Autodesk Inventor part; units mm, degrees
ref_plane "Work Plane1" through (6, 0, -16) normal (0, 0, -1) x (-1, 0, 0)
ref_plane "YZ Plane" through (0, 0, 0) normal (1, 0, 0) x (0, 1, 0)
ref_plane "XZ Plane" through (0, 0, 0) normal (0, 1, 0) x (-1, 0, 0)
sketch "Sketch1" plane through (0, 0, 0) normal (0, 1, 0) x (-1, 0, 0)
  line L0 (6, 8) -> (-6, 8)
  line L1 (-8, 6) -> (-8, -6)
  line L2 (-6, -8) -> (6, -8)
  line L3 (8, -6) -> (8, 6)
  arc A0 (8, 6) -> (6, 8) centre (6, 6) ccw
  arc A1 (-6, 8) -> (-8, 6) centre (-6, 6) ccw
  arc A2 (-8, -6) -> (-6, -8) centre (-6, -6) ccw
  arc A3 (6, -8) -> (8, -6) centre (6, -6) ccw
  point P0 (0, 0)
  point P1 (8, 8)
  point P2 (-8, 8)
  point P3 (8, -8)
  dimension "d0" = 16
  dimension "d1" = 16
  dimension "d2" = 8
  dimension "d3" = 8
  dimension "d4" = 2
extrude "Extrusion1" add sketch "Sketch1" along normal blind 150
sketch "Sketch2" plane through (0, 0, 0) normal (0, -1, 0) x (1, 0, 0)
  line L0 (-6, 5.875) -> (-6, 3.125) construction
  line L1 (-7.375, 5.875) -> (-7.375, 3.125)
  line L2 (-4.625, 3.125) -> (-4.625, 5.875)
  arc A0 (-4.625, 5.875) -> (-7.375, 5.875) centre (-6, 5.875) ccw
  arc A1 (-7.375, 3.125) -> (-4.625, 3.125) centre (-6, 3.125) ccw
  line L3 (6, -3.125) -> (6, -5.875) construction
  line L4 (4.625, -3.125) -> (4.625, -5.875)
  line L5 (7.375, -5.875) -> (7.375, -3.125)
  arc A2 (7.375, -3.125) -> (4.625, -3.125) centre (6, -3.125) ccw
  arc A3 (4.625, -5.875) -> (7.375, -5.875) centre (6, -5.875) ccw
  point P0 (0, 0)
  point P1 (0, 0)
  point P2 (-6, 4.5)
  point P3 (6, -4.5)
  dimension "d7" = 2.75
  dimension "d8" = 12
  dimension "d9" = 6
  dimension "d10" = 9
  dimension "d11" = 4.5
  dimension "d12" = 2.75
  dimension "d13" = 2.75
  dimension "d14" = 2.75
extrude "Extrusion2" cut sketch "Sketch2" against normal blind 2.5
sketch "Sketch3" plane through (0, 150, 0) normal (0, 1, 0) x (1, 0, 0)
  line L0 (-6, 9.5) -> (-6, 6.5) construction
  line L1 (-6.6, 9.5) -> (-6.6, 6.5)
  line L2 (-5.4, 6.5) -> (-5.4, 9.5)
  arc A0 (-5.4, 9.5) -> (-6.6, 9.5) centre (-6, 9.5) ccw
  arc A1 (-6.6, 6.5) -> (-5.4, 6.5) centre (-6, 6.5) ccw
  line L3 (6, 9.5) -> (6, 6.5) construction
  line L4 (5.4, 9.5) -> (5.4, 6.5)
  line L5 (6.6, 6.5) -> (6.6, 9.5)
  arc A2 (6.6, 9.5) -> (5.4, 9.5) centre (6, 9.5) ccw
  arc A3 (5.4, 6.5) -> (6.6, 6.5) centre (6, 6.5) ccw
  line L6 (-6, 8) -> (6, 8) construction
  line L7 (6, 8) -> (-6, 8)
  circle A4 centre (0, 0) radius 3.378 construction
  circle A5 centre (0, 8) radius 3.494
  dimension "d25" = 0.6
  dimension "d26" = 0.6
  dimension "d27" = 3
  dimension "d30" = 12
  dimension "d32" = 3
  dimension "d35" = 6
  dimension "d36" = 0
extrude "Extrusion3" add sketch "Sketch3" along normal blind 1.5 contours A0 L2 A1 L1 | L4 A2 L5 A3
ref_plane "Work Plane1" through (6, 0, -16) normal (0, 0, -1) x (-1, 0, 0)
sketch "Sketch4" plane through (6, 0, -16) normal (0, 0, -1) x (-1, 0, 0)
  line L0 (-2, 0) -> (-2, 150)
  line L1 (14, 0) -> (14, 150)
  line L2 (-2, 150) -> (14, 150)
  line L3 (14, 150) -> (14, 135)
  line L4 (14, 135) -> (-2, 135)
  line L5 (-2, 135) -> (-2, 150)
  point P0 (6, 0)
  dimension "d38" = 15
extrude "Extrusion4" add sketch "Sketch4" against normal blind 10
fillet "Fillet1" radius 2 2 edges at (8, 142.5, -16) (-8, 142.5, -16)
sketch "Sketch5" plane through (8, 0, 6) normal (1, 0, 0) x (0, 0, -1)
  line L0 (22, 135) -> (22, 150)
  line L1 (22, 146) -> (6, 146)
  line L2 (6, 146) -> (6, 20)
  line L3 (6, 20) -> (22, 20)
  line L4 (22, 20) -> (22, 146)
  line L5 (-2, 0) -> (-2, 150)
  line L6 (0, 150) -> (20, 150)
  point P0 (6, 0)
  dimension "d42" = 8
  dimension "d43" = 20
  dimension "d44" = 4
extrude "Extrusion5" cut sketch "Sketch5" against normal up to surface (16 mm away)
hole "Hole2" at (0, 150, -8) direction (0, -1, 0) diameter 6.756 depth 7
sketch "Sketch6" plane through (8, 0, 6) normal (1, 0, 0) x (0, 0, -1)
  line L0 (22, 146) -> (20, 146)
  arc A0 (22, 146) -> (6, 109.9866) centre (54.5302, 109.9866) ccw
  line L1 (20, 146) -> (6, 146)
  line L2 (6, 109.9866) -> (6, 146)
  line L3 (6, 146) -> (22, 146)
  point P0 (6, 0)
extrude "Extrusion6" add sketch "Sketch6" against normal up to surface (16 mm away)
sketch "Sketch7" plane through (0, 150, 0) normal (0, 1, 0) x (1, 0, 0)
  circle A0 centre (0, 8) radius 3.378 construction
  arc A1 (-6, 16) -> (-8, 14) centre (-6, 14) ccw
  line L0 (-8, 14) -> (-8, -6)
  arc A2 (-8, -6) -> (-6, -8) centre (-6, -6) ccw
  line L1 (-6, -8) -> (6, -8)
  arc A3 (6, -8) -> (8, -6) centre (6, -6) ccw
  line L2 (8, -6) -> (8, 14)
  arc A4 (8, 14) -> (6, 16) centre (6, 14) ccw
  line L3 (6, 16) -> (-6, 16)
  line L4 (6.6, 6.5) -> (6.6, 9.5) construction
  arc A5 (5.4, 6.5) -> (6.6, 6.5) centre (6, 6.5) ccw construction
  line L5 (5.4, 9.5) -> (5.4, 6.5) construction
  arc A6 (6.6, 9.5) -> (5.4, 9.5) centre (6, 9.5) ccw construction
  line L6 (-6.6, 9.5) -> (-6.6, 6.5) construction
  arc A7 (-5.4, 9.5) -> (-6.6, 9.5) centre (-6, 9.5) ccw construction
  line L7 (-5.4, 9.5) -> (-5.4, 6.5) construction
  arc A8 (-6.6, 6.5) -> (-5.4, 6.5) centre (-6, 6.5) ccw construction
  line L8 (-17.4625, -22.225) -> (15.875, -22.225)
  line L9 (15.875, -22.225) -> (15.875, 22.225)
  line L10 (15.875, 22.225) -> (-17.4625, 22.225)
  line L11 (-17.4625, 22.225) -> (-17.4625, -22.225)
  point P0 (0, 0)
extrude "Extrusion7" cut sketch "Sketch7" against normal blind 10
sketch "Sketch8" plane through (6, 0, -16) normal (0, 0, -1) x (-1, 0, 0)
  line L0 (0, 146) -> (12, 146)
  line L1 (14, 109.9866) -> (-2, 109.9866)
  line L2 (0, 146) -> (12, 146)
  line L3 (12, 146) -> (12, 109.9866)
  line L4 (12, 109.9866) -> (0, 109.9866)
  line L5 (0, 109.9866) -> (0, 146)
  line L6 (-2, 109.9866) -> (-2, 144.0871)
  line L7 (14, 109.9866) -> (14, 144.0871)
  point P0 (6, 0)
  dimension "d68" = 2
  dimension "d69" = 2
extrude "Extrusion8" cut sketch "Sketch8" against normal up to surface (16 mm away)
hole "Hole3" at (0, 0, 0) direction (0, 1, 0) diameter 5.4 depth 40
equation "\"d12\" = d7"
equation "\"d13\" = d7"
equation "\"d14\" = d7"
equation "\"d26\" = d25"
equation "\"d27\" = d32"
equation "\"d35\" = 0.5 * d30"
equation "\"d69\" = d68"
properties part number "Camera Mount 30mm"
Work out the finished part from the listing and answer in its coordinate system (mm). A direction names the side the tool comes from. Give positions to 0.01 mm unless a question says otherwise; leave off trailing zeros. Loops run counter-clockwise (first coordinate to the right, second up) from the corner with the lowest first, then second, coordinate; pieces in that order, holes last. Notation, with made-up numbers: (31, 25) - (56, 25) arc R16 cw to (56, 29) - close; hole circle Ø1 at (75.25, 12). An arc over 180 degrees is marked (long way). Answer in a Markdown table with one row per item.
(1) Flat-ended cylindrical pins translate along their axes: pin 1 Ø5 at (x, y) = (-2, 111.5) entering from -Z; pin 2 Ø0.8 at (x, z) = (-6.5, 5.5) entering from -Y; pin 3 Ø8 at (x, z) = (5, 1.5) entering from +Y; pin 4 Ø13 at (y, z) = (130.5, -8) entering from +X. Find the tip coordinate at first contact, or state that the pin passes through.
Results list:
| item | result |
|---|---|
| pin 1 | stops at z = 0 |
| pin 2 | stops at y = 2.5 |
| pin 3 | stops at y = 150 |
| pin 4 | stops at x = 8 |
(2) Section A-A (x = 0) is taken. Give the vertices of the cut face in (y, z), and give its area (3 significant figures).
Results list:
| item | result |
|---|---|
| outline | (0, -8) - (20, -8) - (20, -2.7) - (0, -2.7) - close; (0, 2.7) - (40, 2.7) - (40, 0) - (146, 0) - (146, -4.62) - (150, -4.62) - (150, 8) - (0, 8) - close; (146, -16) - (150, -16) - (150, -11.38) - (146, -11.38) - close |
| area | 1,230 mm² |
(3) Section B-B (y = 29.5) is taken. Give the vertices of the cut face in (x, z), and give its area (3 significant figures).
Results list:
| item | result |
|---|---|
| outline | (-8, 0) - (-2.7, 0) arc R2.7 cw to (2.7, 0) - (8, 0) - (8, 6) arc R2 ccw to (6, 8) - (-6, 8) arc R2 ccw to (-8, 6) - close |
| area | 115 mm² |
(4) A tool of negligible diameter and unlimited length cuts with its end or side. For faces 1 (the face through (7.375, 1, -5)), 2 (the face through (6, 137, -5)), 3 (the face through (0, 10, -8)), 4 (the face through (8, 76, 1)), 5 (the face through (7.014, 129.95, -4.296)), from which of +Z, -Z, +X, -X, +Y, -Y can it reach the whole face along a straight path? Write none if from no direction.
Results list:
| item | result |
|---|---|
| face 1 | -Y |
| face 2 | -Z |
| face 3 | -Z, +X, -X, -Y |
| face 4 | +Z, -Z, +X, +Y, -Y |
| face 5 | -Z, +X, -X |
(5) For a pull along X with two mould halves and no side action, classify faces 6 (the face through (6, 2.5, -4)), 7 (the face through (0, 148, -16)), 8 (the face through (-8, 76, 1)) as pulls with the +X half, pulls with the -X half, needs draft (parallel to the pull), parting line crosses it, or undercut.
Results list:
| item | result |
|---|---|
| face 6 | undercut |
| face 7 | needs draft |
| face 8 | pulls with the -X half |
(6) Section C-C (y = 101) is taken. Give the vertices of the cut face in (x, z).
Results list:
| item | result |
|---|---|
| outline | (-8, 0) - (8, 0) - (8, 6) arc R2 ccw to (6, 8) - (-6, 8) arc R2 ccw to (-8, 6) - close |
(7) Consider L1, parallel to Z at x = 0, y = 9; L2, parallel to Z at x = 0, y = 148.8; L3, parallel to X at y = 148.65, z = -8. Determine where each line is inside the solid, lowest interval first. Write a range as [from, to].
Results list:
| item | result |
|---|---|
| L1 | z = [-8, -2.7], [2.7, 8] |
| L2 | z = [-16, -11.38], [-4.62, 8] |
| L3 | x = [-8, -3.38], [3.38, 8] |
